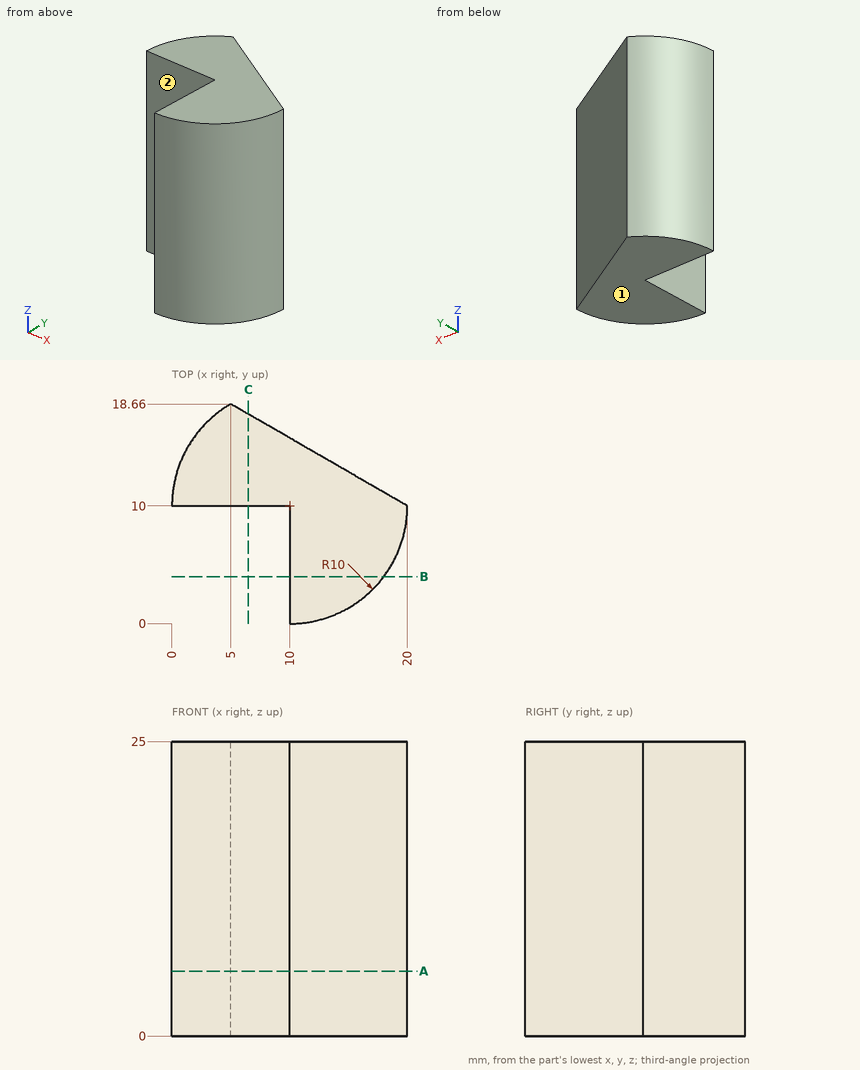
Study the drawing (mm; zero at the part's minimum x, y, z) and answer. A direction names the side the tool comes from. Give positions to 0.01 mm unless a question says otherwise; leave off trailing zeros. Order: outer loops, then holes, each group sorted by start corner. A loop starts at its lowest first (then second) coordinate and runs counter-clockwise, first axis right, second up.
1) Consider line 1 along Y through (x, z) = (7.5, 14.75); line 2 along X through (y, z) = (16, 19.25); line 3 along Y through (x, z) = (16.25, 14.5) (1 decimal). Determine where each line is inside the solid, lowest interval first.
Reported:
line 1: y = 10 to 17.22
line 2: x = 2 to 9.61
line 3: y = 2.2 to 12.2
2) Given P1, Ø8, axis at y = 15, z = 7, coming from the +X side; P2, Ø1.5, axis at y = 6, z = 10.5, coming from the +X side; P3, Ø1.5, axis at x = 5.5, z = 7.5, coming from the +Y side; P4, Ø1.5, axis at x = 9, y = 7.5, coming from the +Z side, each flat-ended and moving along its own axis, determine where each tip first touches the part or whether it passes through.
Reported:
P1: stops at x = 18.27
P2: stops at x = 19.46
P3: stops at y = 18.66
P4: passes through
3) Find section C-C on x = 6.5. Write down the section's boundary in (y, z), then the cut area to 3 significant figures.
Reported:
outline: (10, 0) - (17.79, 0) - (17.79, 25) - (10, 25) - close
area: 195 mm2
4) Find section B-B on y = 4. Write down the section's boundary in (x, z).
Reported:
outline: (10, 0) - (18, 0) - (18, 25) - (10, 25) - close
5) For the marked faces 1 and 2, determine the directions among +Z, -Z, +X, -X, +Y, -Y from which every point of the face is accessible in a straight line to the end or side of a thin tool.
Reported:
face 1: -Z, +X, -X, +Y, -Y
face 2: +Z, -Z, -X, -Y
6) Find section A-A on z = 5.5. Write down the section's boundary in (x, y).
Reported:
outline: (0, 10) - (10, 10) - (10, 0) arc R10 ccw to (20, 10) - (5, 18.66) arc R10 ccw to start
